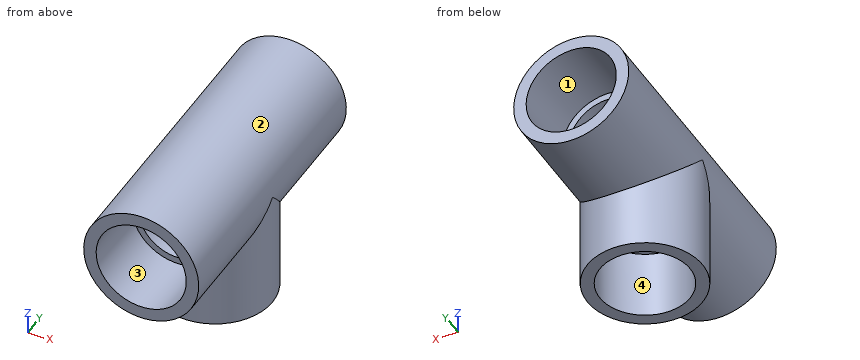
from build123d import *

# Parameters (mm, degrees)
SKETCH1_R           = 17.145
SKETCH1_R_2         = 11.43
BOSS_EXTRUDE1_DEPTH = 84.328
SKETCH2_R           = 17.145
SKETCH2_R_2         = 11.43
BOSS_EXTRUDE2_DEPTH = 35.56
SKETCH3_R           = 11.43
CUT_EXTRUDE1_DEPTH  = 94.111096186
CUT_EXTRUDE2_START  = -35.56
SKETCH4_R           = 11.43
CUT_EXTRUDE2_DEPTH  = 35.56
SKETCH5_R           = 13.4366
CUT_EXTRUDE3_DEPTH  = 20.6375
CUT_EXTRUDE4_START  = -20.6375
SKETCH6_R           = 13.4366
CUT_EXTRUDE4_DEPTH  = 20.6375
SKETCH7_R           = 13.4366
CUT_EXTRUDE5_DEPTH  = 20.6375


with BuildPart() as part:
    # Sketch1 → Boss-Extrude1 (new body)
    with BuildSketch(Plane(origin=(0, 0, 0), x_dir=(1, 0, 0), z_dir=(0, 1, 0))):
        with Locations(Location((0, 0, 0), (0, 0, 270))):
            Circle(SKETCH1_R)
        with Locations(Location((0, 0, 0), (0, 0, 270))):
            Circle(SKETCH1_R_2, mode=Mode.SUBTRACT)
    extrude(amount=BOSS_EXTRUDE1_DEPTH)

    # Sketch2 → Boss-Extrude2 (add)
    with BuildSketch(Plane.XY):
        with Locations((0, 42.164)):
            Circle(SKETCH2_R)
        with Locations((0, 42.164)):
            Circle(SKETCH2_R_2, mode=Mode.SUBTRACT)
    extrude(amount=-BOSS_EXTRUDE2_DEPTH)

    # Sketch3 → Cut-Extrude1 (cut, through all)
    with BuildSketch(Plane(origin=(0, 84.328, 0), x_dir=(1, 0, 0), z_dir=(0, 1, 0))):
        with Locations(Location((0, 0, 0), (0, 0, 270))):
            Circle(SKETCH3_R)
    extrude(amount=-CUT_EXTRUDE1_DEPTH, mode=Mode.SUBTRACT)

    # Sketch4 → Cut-Extrude2 (cut)
    with BuildSketch(Plane(origin=(0, 0, -35.56), x_dir=(-1, 0, 0), z_dir=(0, 0, -1)).offset(CUT_EXTRUDE2_START)):
        with Locations(Location((0, 42.164, 0), (0, 0, 180))):
            Circle(SKETCH4_R)
    extrude(amount=CUT_EXTRUDE2_DEPTH, mode=Mode.SUBTRACT)

    # Sketch5 → Cut-Extrude3 (cut)
    with BuildSketch(Plane(origin=(0, 84.328, 0), x_dir=(1, 0, 0), z_dir=(0, 1, 0))):
        with Locations(Location((0, 0, 0), (0, 0, 270))):
            Circle(SKETCH5_R)
    extrude(amount=-CUT_EXTRUDE3_DEPTH, mode=Mode.SUBTRACT)

    # Sketch6 → Cut-Extrude4 (cut)
    with BuildSketch(Plane.XZ.offset(CUT_EXTRUDE4_START)):
        with Locations(Location((0, 0, 0), (0, 0, 90))):
            Circle(SKETCH6_R)
    extrude(amount=CUT_EXTRUDE4_DEPTH, mode=Mode.SUBTRACT)

    # Sketch7 → Cut-Extrude5 (cut)
    with BuildSketch(Plane(origin=(0, 0, -35.56), x_dir=(-1, 0, 0), z_dir=(0, 0, -1))):
        with Locations((0, 42.164)):
            Circle(SKETCH7_R)
    extrude(amount=-CUT_EXTRUDE5_DEPTH, mode=Mode.SUBTRACT)


solid = part.part
For this review, take the finished solid that the model builds, in its own axes (mm). Face numbers are marked on the shaded views. Give positions to 0.01 mm unless a question says otherwise; leave off trailing zeros. Loops run counter-clockwise (first coordinate to the right, second up) from the corner with the lowest first, then second, coordinate; pieces in that order, holes last. Notation, with made-up numbers: M -5,8 L 22,8 A16 cw 22,13 Z; hole C -20,45.5 d11. An arc over 180 degrees is marked long. Answer as a JSON object with one key per item and string values. Group by question number.
Q1. Add section B-B on z = -10. Give the boundary of the cut face in (x, y) (1 decimal).
Q2. Add section C-C on y = 72.5. Give the boundary of the cut face in (x, z) (3 decimals).
Q3. Mouldability with a two-part tool opening along Z and no side actions: class the marked faces 1, 2, 3 and 4 as +Z half, -Z half, draft (parallel to the pull), parting line (faces both ways), or undercut.
Q4. For probe 1 along X at (y, z) = (69.5, 0) (3 decimals); probe 2 along Y at (x, z) = (0, -24); probe 3 along X at (y, z) = (45, -25), list the stretches that pass through material, from the lowest coordinate up. Write a range as [from, to].
Q5. Add section A-A on x = 0. Give the boundary of the cut face in (y, z) (1 decimal), and give its area (3 significant figures).
Q6. Add section D-D on x = 15. Give the boundary of the cut face in (y, z), and give its area (3 significant figures).
Q7. Insertion check: P1, Ø8, axis at x = 5.5, y = 38.5, coming from the -Z side; P2, Ø10, axis at x = -2.5, z = -28.5, coming from the -Y side; P3, Ø6, axis at y = 38.5, z = -15, coming from the -X side; P4, Ø18.5, axis at x = 0, z = 0, coming from the +Y side. Each pin has a flat end and moves straight along its axis. Give the tip position at first contact, or say it passes through.
Checked values:
{
 "1": {"outline": "M -13.9,0 L -9,0 L -9,20.6 L -5.5,20.6 L -5.5,32.2 A11.4 cw -5.5,52.2 L -5.5,63.7 L -9,63.7 L -9,84.3 L -13.9,84.3 L -13.9,52.2 A17.1 ccw -13.9,32.2 Z; M 5.5,20.6 L 9,20.6 L 9,0 L 13.9,0 L 13.9,32.2 A17.1 ccw 13.9,52.2 L 13.9,84.3 L 9,84.3 L 9,63.7 L 5.5,63.7 L 5.5,52.2 A11.4 cw 5.5,32.2 Z"},
 "2": {"outline": "C 0,0 d34.29; hole C 0,0 d26.873"},
 "3": {"face 1": "undercut", "face 2": "parting line", "face 3": "undercut", "face 4": "draft"},
 "4": {"probe 1": "[-17.145, -13.437], [13.437, 17.145]", "probe 2": "[25.02, 28.73], [55.6, 59.31]", "probe 3": "[-16.91, -13.13], [13.13, 16.91]"},
 "5": {"outline": "M 0,-17.1 L 25,-17.1 L 25,-35.6 L 28.7,-35.6 L 28.7,-14.9 L 30.7,-14.9 L 30.7,-11.4 L 20.6,-11.4 L 20.6,-13.4 L 0,-13.4 Z; M 0,13.4 L 20.6,13.4 L 20.6,11.4 L 63.7,11.4 L 63.7,13.4 L 84.3,13.4 L 84.3,17.1 L 0,17.1 Z; M 53.6,-14.9 L 55.6,-14.9 L 55.6,-35.6 L 59.3,-35.6 L 59.3,-17.1 L 84.3,-17.1 L 84.3,-13.4 L 63.7,-13.4 L 63.7,-11.4 L 53.6,-11.4 Z", "area": "795 mm²"},
 "6": {"outline": "M 0,-8.3 L 33.86,-8.3 L 33.86,-35.56 L 50.47,-35.56 L 50.47,-8.3 L 84.33,-8.3 L 84.33,8.3 L 0,8.3 Z", "area": "1,850 mm²"},
 "7": {"P1": "z = 6.36", "P2": "y = 25.02", "P3": "x = -17.13", "P4": "through"}
}
